```python
from build123d import *

# Parameters (mm, degrees)
SKETCH1_W           = 150
SKETCH1_H           = 70
SKETCH1_R           = 25
SKETCH1_R_2         = 20
BOSS_EXTRUDE1_DEPTH = 10
BOSS_EXTRUDE2_START = 10
SKETCH1_3_R         = 25
SKETCH1_3_R_2       = 20
BOSS_EXTRUDE2_DEPTH = 40
SKETCH6_R           = 3
CUT_EXTRUDE1_DEPTH  = 11


with BuildPart() as part:
    # Sketch1 → Boss-Extrude1 (new body)
    with BuildSketch(Plane.XY):
        Rectangle(SKETCH1_W, SKETCH1_H)
        Circle(SKETCH1_R, mode=Mode.SUBTRACT)
        Circle(SKETCH1_R)
        Circle(SKETCH1_R_2, mode=Mode.SUBTRACT)
    extrude(amount=BOSS_EXTRUDE1_DEPTH)

    # Sketch1<3> → Boss-Extrude2 (add)
    with BuildSketch(Plane.XY.offset(BOSS_EXTRUDE2_START)):
        Circle(SKETCH1_3_R)
        Circle(SKETCH1_3_R_2, mode=Mode.SUBTRACT)
    extrude(amount=BOSS_EXTRUDE2_DEPTH)

    # Sketch6 → Cut-Extrude1 (cut, through all)
    with BuildSketch(Plane.XY.offset(10)):
        with Locations((-65, 20)):
            Circle(SKETCH6_R)
        with Locations((-65, -20)):
            Circle(SKETCH6_R)
        with Locations((65, -20)):
            Circle(SKETCH6_R)
        with Locations((65, 20)):
            Circle(SKETCH6_R)
    extrude(amount=-CUT_EXTRUDE1_DEPTH, mode=Mode.SUBTRACT)


solid = part.part
```
Model file for the job. Use its own axes, mm. A direction names the side the tool comes from. Coordinates: 2 decimals unless noted, no trailing zeros. Write each loop counter-clockwise with the first axis right and the second up, starting at its lowest first coordinate (ties: lowest second). Pieces come first, ordered by that corner, then holes. Notation, with made-up numbers: (11.25, -4) - (30.25, -4) arc R33 cw to (30.25, 31) - close; hole circle Ø1 at (3, 32.25). An arc over 180 degrees is marked (long way). Use a Markdown table: item, result. Add a question column.
Item 1: Drill centre lines: line 1 along Y through (x, z) = (65, 5.75); line 2 along Y through (x, z) = (1, 22); line 3 along Z through (x, y) = (-36, 15). Where is each one in solid material? Low to high.
Item 2: Drop flat-ended pins along their axis: pin 1 (1 mm diameter, centred on y = 22.5, z = 42, fed in from -X); pin 2 (4 mm diameter, centred on y = -7.5, z = 38.5, fed in from -X); pin 3 (6 mm diameter, centred on x = -19.5, z = 21, fed in from -Y). Give the stop position or say it passes through.
Item 3: Two-plate mould, pull along X, no slides. Class faces 1 (the face through (62, -20, 5)), 2 (the face through (-67.4, 18.2, 5.1)), 3 (the face through (-1, -35, 5)), 4 (the face through (75, 0, 5)): pulls with the +X half, pulls with the -X half, needs draft (parallel to the pull), parting line crosses it, or undercut.
Item 4: Band-saw the part on C-C, the plane x = 5.5. Write the cut outline in (y, z), and give its area (3 significant figures).
Item 5: Band-saw the part on B-B, the plane x = -65. Write the cut outline in (y, z).
Item 6: 3-axis set-ups, long thin cutter, end or side, ignore diameter. For faces 5 (the face through (23.846, 7.509, 29.72)), 6 (the face through (-4.336, -19.524, 24.65)): which of +Z, -Z, +X, -X, +Y, -Y reach the whole face in a straight line?
Item 7: Band-saw the part on D-D, the plane z = 35.5. Write the cut outline in (x, y).
Item 8: Band-saw the part on A-A, the plane y = 0. Write the cut outline in (x, z), and give its area (3 significant figures).
A:
| question | item | result |
|---|---|---|
| 1 | line 1 | y = -35 to -23, -17 to 17, 23 to 35 |
| 1 | line 2 | y = -24.98 to -19.97, 19.97 to 24.98 |
| 1 | line 3 | z = 0 to 10 |
| 2 | pin 1 | stops at x = -11.87 |
| 2 | pin 2 | stops at x = -24.39 |
| 2 | pin 3 | stops at y = -18.78 |
| 3 | face 1 | undercut |
| 3 | face 2 | undercut |
| 3 | face 3 | needs draft |
| 3 | face 4 | pulls with the +X half |
| 4 | outline | (-35, 0) - (-19.23, 0) - (-19.23, 50) - (-24.39, 50) - (-24.39, 10) - (-35, 10) - close; (19.23, 0) - (35, 0) - (35, 10) - (24.39, 10) - (24.39, 50) - (19.23, 50) - close |
| 4 | area | 728 mm² |
| 5 | outline | (-35, 0) - (-23, 0) - (-23, 10) - (-35, 10) - close; (-17, 0) - (17, 0) - (17, 10) - (-17, 10) - close; (23, 0) - (35, 0) - (35, 10) - (23, 10) - close |
| 6 | face 5 | +Z |
| 6 | face 6 | +Z, -Z |
| 7 | outline | circle Ø50 at (0, 0); hole circle Ø40 at (0, 0) |
| 8 | outline | (-75, 0) - (-20, 0) - (-20, 50) - (-25, 50) - (-25, 10) - (-75, 10) - close; (20, 0) - (75, 0) - (75, 10) - (25, 10) - (25, 50) - (20, 50) - close |
| 8 | area | 1,500 mm² |
